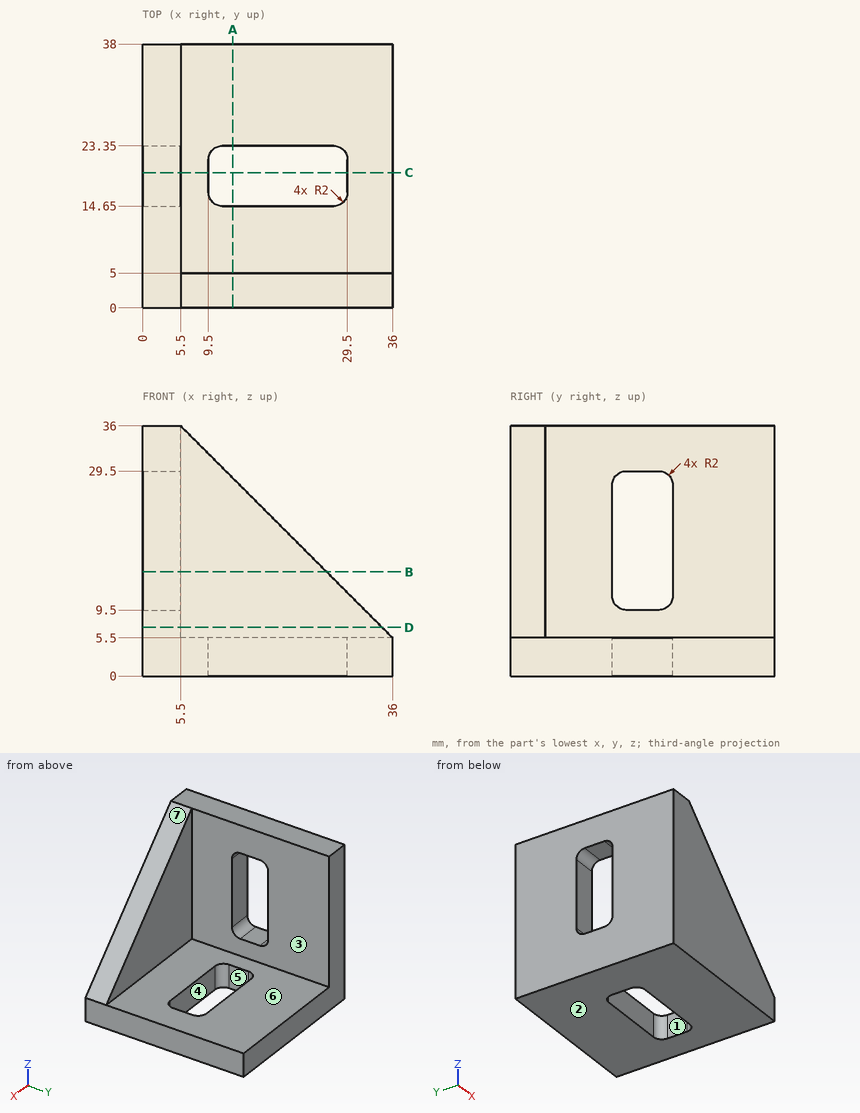
Input: dimensioned drawing with shaded views. Units: mm. Origin: part minimum x, y, z. A direction names the side the tool comes from. Round coordinates to 2 decimals unless told otherwise and drop trailing zeros. Order: outer loops, then holes, each group sorted by start corner. A loop starts at its lowest first (then second) coordinate and runs counter-clockwise, first axis right, second up. Notation, with made-up numbers: (59, -31.5) -> (83, -31.5) arc R14 ccw to (83, -8.5) -> close; hole circle Ø6 at (43, 54). An arc over 180 degrees is marked (long way). Put each result on its own line as item: value. Start each with the question number.
Q1. Line query: probe 1 along Y at (x, z) = (26, 4); probe 2 along Z at (x, y) = (20, 26); probe 3 along X at (y, z) = (21, 1.5). Output: solid intervals per line, ascending.
Q2. First-contact query: pin 1 (1 mm diameter, centred on x = 12, y = 21, fed in from -Z); pin 2 (9 mm diameter, centred on y = 16, z = 27.5, fed in from +X). Flat tips, straight axial feed; report the tip coordinate or a pass-through.
Q3. Section D-D on z = 7. Return the cut outline in (x, y), and give its area (3 significant figures).
Q4. Section C-C on y = 19.5. Return the cut outline in (x, z).
Q5. Reachability of the marked faces 5, 6 and 7 from +Z, -Z, +X, -X, +Y, -Y: full face, straight path, thin tool, end or side. Return the list, or none.
Q6. Section B-B on z = 15. Return the cut outline in (x, y).
Q7. Section A-A on x = 13. Return the cut outline in (y, z).
Q8. Pull-direction query (X, two-part tool) for the marked faces 1, 2, 3 and 4; classes: +X half, -X half, draft (parallel to the pull), parting line (faces both ways), or undercut.
Ans:
1. probe 1: y = 0 to 14.65, 23.35 to 38
1. probe 2: z = 0 to 5.5
1. probe 3: x = 0 to 9.5, 29.5 to 36
2. pin 1: passes through
2. pin 2: stops at x = 5.5
3. outline: (0, 0) -> (34.5, 0) -> (34.5, 5) -> (5.5, 5) -> (5.5, 38) -> (0, 38) -> close
3. area: 354 mm2
4. outline: (0, 0) -> (9.5, 0) -> (9.5, 5.5) -> (5.5, 5.5) -> (5.5, 9.5) -> (0, 9.5) -> close; (0, 29.5) -> (5.5, 29.5) -> (5.5, 36) -> (0, 36) -> close; (29.5, 0) -> (36, 0) -> (36, 5.5) -> (29.5, 5.5) -> close
5. face 5: +Z, -Z
5. face 6: +Z, +X, +Y
5. face 7: +Z, +X, +Y, -Y
6. outline: (0, 0) -> (26.5, 0) -> (26.5, 5) -> (5.5, 5) -> (5.5, 14.65) -> (0, 14.65) -> close; (0, 23.35) -> (5.5, 23.35) -> (5.5, 38) -> (0, 38) -> close
7. outline: (0, 0) -> (14.65, 0) -> (14.65, 5.5) -> (5, 5.5) -> (5, 28.5) -> (0, 28.5) -> close; (23.35, 0) -> (38, 0) -> (38, 5.5) -> (23.35, 5.5) -> close
8. face 1: undercut
8. face 2: draft
8. face 3: +X half
8. face 4: undercut
